from build123d import *

# Parameters (mm, degrees)
SKETCH1_W           = 30.5
SKETCH1_H           = 85
BOSS_EXTRUDE1_DEPTH = 2
CUT_EXTRUDE1_DEPTH  = 2
SKETCH5_W           = 0.8
SKETCH5_H           = 4
BOSS_EXTRUDE2_DEPTH = 3
SKETCH6_R           = 1
CUT_EXTRUDE2_DEPTH  = 0.8
FILLET1_R           = 2
FILLET2_R           = 2
SKETCH7_W           = 30.5
SKETCH7_H           = 2
BOSS_EXTRUDE3_DEPTH = 16
SKETCH8_W           = 30.5
SKETCH8_H           = 80
BOSS_EXTRUDE4_DEPTH = 1.8
SKETCH9_W           = 28.5
SKETCH9_H           = 80
CUT_EXTRUDE3_DEPTH  = 1.8
SKETCH10_W          = 28.9
SKETCH10_H          = 2
CUT_EXTRUDE4_DEPTH  = 1
SKETCH11_W          = 7
SKETCH11_H          = 6
CUT_EXTRUDE5_DEPTH  = 2


with BuildPart() as part:
    # Sketch1 → Boss-Extrude1 (new body)
    with BuildSketch(Plane(origin=(0, 0, 0), x_dir=(1, 0, 0), z_dir=(0, 1, 0))):
        Rectangle(SKETCH1_W, SKETCH1_H)
    extrude(amount=BOSS_EXTRUDE1_DEPTH)

    # Sketch2 → Cut-Extrude1 (cut)
    with BuildSketch(Plane(origin=(0, 2, 0), x_dir=(1, 0, 0), z_dir=(0, 1, 0))):
        Polygon((14.45, 42.5), (-14.45, 42.5), (-14.45, 24.5), (-14.45, 22.5), (14.45, 22.5), (14.45, 24.5), align=None)
    extrude(amount=-CUT_EXTRUDE1_DEPTH, mode=Mode.SUBTRACT)

    # Sketch5 → Boss-Extrude2 (add)
    with BuildSketch(Plane(origin=(0, 2, 0), x_dir=(1, 0, 0), z_dir=(0, 1, 0))):
        with Locations((-14.85, 40.5)):
            Rectangle(SKETCH5_W, SKETCH5_H)
    boss_extrude2 = extrude(amount=BOSS_EXTRUDE2_DEPTH)

    # Sketch6 → Cut-Extrude2 (cut)
    with BuildSketch(Plane.ZY.offset(15.25)):
        with Locations((-40.5, 2)):
            Circle(SKETCH6_R)
    cut_extrude2 = extrude(amount=-CUT_EXTRUDE2_DEPTH, mode=Mode.SUBTRACT)

    # Mirror1: Boss-Extrude2, Cut-Extrude2 across plane
    add(boss_extrude2.mirror(Plane(origin=(0, 0, 0), x_dir=(0, 0, 1), z_dir=(1, 0, 0))))
    add(cut_extrude2.mirror(Plane(origin=(0, 0, 0), x_dir=(0, 0, 1), z_dir=(1, 0, 0))), mode=Mode.SUBTRACT)

    # Fillet1
    fillet1_edges = [part.edges().sort_by_distance(p)[0] for p in [
        (-14.85, 0, -42.5),
        (-14.85, 5, -42.5),
        (-14.85, 5, -38.5),
    ]]
    fillet(fillet1_edges, radius=FILLET1_R - 0.0001)  # a hair under: the kernel refuses the full size

    # Fillet2
    fillet2_edges = [part.edges().sort_by_distance(p)[0] for p in [
        (14.85, 0, -42.5),
        (14.85, 5, -38.5),
        (14.85, 5, -42.5),
    ]]
    fillet(fillet2_edges, radius=FILLET2_R - 0.0001)  # a hair under: the kernel refuses the full size

    # Sketch7 → Boss-Extrude3 (add)
    with BuildSketch(Plane.XY.offset(42.5)):
        with Locations((0, 1)):
            Rectangle(SKETCH7_W, SKETCH7_H)
    extrude(amount=BOSS_EXTRUDE3_DEPTH)

    # Sketch8 → Boss-Extrude4 (add)
    with BuildSketch(Plane(origin=(0, 2, 0), x_dir=(1, 0, 0), z_dir=(0, 1, 0))):
        with Locations((0, -18.5)):
            Rectangle(SKETCH8_W, SKETCH8_H)
    extrude(amount=BOSS_EXTRUDE4_DEPTH)

    # Sketch9 → Cut-Extrude3 (cut)
    with BuildSketch(Plane(origin=(0, 3.8, 0), x_dir=(1, 0, 0), z_dir=(0, 1, 0))):
        with Locations((0, -18.5)):
            Rectangle(SKETCH9_W, SKETCH9_H)
    extrude(amount=-CUT_EXTRUDE3_DEPTH, mode=Mode.SUBTRACT)

    # Sketch10 → Cut-Extrude4 (cut)
    with BuildSketch(Plane(origin=(0, 0, -22.5), x_dir=(-1, 0, 0), z_dir=(0, 0, -1))):
        with Locations((0, 1)):
            Rectangle(SKETCH10_W, SKETCH10_H)
    extrude(amount=-CUT_EXTRUDE4_DEPTH, mode=Mode.SUBTRACT)

    # Sketch11 → Cut-Extrude5 (cut)
    with BuildSketch(Plane(origin=(0, 2, 0), x_dir=(1, 0, 0), z_dir=(0, 1, 0))):
        with Locations((10.75, -50.5)):
            Rectangle(SKETCH11_W, SKETCH11_H)
    extrude(amount=-CUT_EXTRUDE5_DEPTH, mode=Mode.SUBTRACT)


solid = part.part
For this review, take the finished solid that the model builds, in its own axes (mm). A direction names the side the tool comes from. Give positions to 0.01 mm unless a question says otherwise; leave off trailing zeros. Order: outer loops, then holes, each group sorted by start corner. A loop starts at its lowest first (then second) coordinate and runs counter-clockwise, first axis right, second up. Notation, with made-up numbers: (8.25, -33.5) - (25.25, -33.5) arc R20 cw to (25.25, -12.5) - close; hole circle Ø3 at (23, 2). An arc over 180 degrees is marked (long way). Answer as a JSON object with one key per item and string values. Group by question number.
Item 1: Clearance check with flat-ended pins moving along their axes: pin 1 Ø1.6 at (x, y) = (10, 1.5) entering from -Z; pin 2 Ø0.8 at (x, z) = (14.5, 29) entering from +Y; pin 3 Ø3 at (x, z) = (12, 5) entering from -Y; pin 4 Ø1.6 at (y, z) = (2, -40.5) entering from -X. State where each tip first meets the part, or that it passes through.
Item 2: Take a section at C-C on x = 1.5. Give the boundary of the cut face in (y, z), and give its area (3 significant figures).
Item 3: Draft analysis for pull direction Z (two halves, no side actions). For faces 1 (the flat face through (0, 2, 18)), 2 (the cylindrical face through (-14.84, 4.4, -39.07)), 3 (the cylindrical face through (-14.84, 0.57, -41.9)), 4 (the flat face through (11, 1, 53.5)), state which applies: pulls with the +Z half, pulls with the -Z half, needs draft (parallel to the pull), parting line crosses it, or undercut.
Item 4: Machinability: for faces 5 (the flat face through (-14.25, 3, 19)), 6 (the flat face through (15.25, 2, 9)), 7 (the flat face through (11, 1, 47.5)), 8 (the flat face through (-14.45, 1, -32)), which of the approach directions +Z, -Z, +X, -X, +Y, -Y give a long, thin tool a straight path to every point of the face, cutting with its end or side? Answer none if there is none.
Item 5: Take a section at B-B on z = -3. Give the boundary of the cut face in (x, y), and give its area (3 significant figures).
Item 6: Take a section at A-A on z = -31.5. Give the boundary of the cut face in (x, y).
Item 7: Wall thickness on line 1 along Y through (x, z) = (-14.8, -40.5); line 2 along X through (y, z) = (2.35, 31); line 3 along Z through (x, y) = (14, 0.2): over which ranges is each line inside the solid? List them lowest first.
Reported:
{
 "1": {"pin 1": "z = -21.5", "pin 2": "y = 3.8", "pin 3": "y = 0", "pin 4": "through"},
 "2": {"outline": "(0, -21.5) - (2, -21.5) - (2, 58.5) - (0, 58.5) - close", "area": "160 mm^2"},
 "3": {"face 1": "needs draft", "face 2": "undercut", "face 3": "pulls with the -Z half", "face 4": "undercut"},
 "4": {"face 5": "+Z, -Z, +Y", "face 6": "+Z, -Z, +X, +Y, -Y", "face 7": "+Y, -Y", "face 8": "-Z, +Y, -Y"},
 "5": {"outline": "(-15.25, 0) - (15.25, 0) - (15.25, 3.8) - (14.25, 3.8) - (14.25, 2) - (-14.25, 2) - (-14.25, 3.8) - (-15.25, 3.8) - close", "area": "64.6 mm^2"},
 "6": {"outline": "(-15.25, 0) - (-14.45, 0) - (-14.45, 2) - (-15.25, 2) - close; (14.45, 0) - (15.25, 0) - (15.25, 2) - (14.45, 2) - close"},
 "7": {"line 1": "0 to 1, 3 to 5", "line 2": "-15.25 to -14.25, 14.25 to 15.25", "line 3": "-21.5 to 47.5, 53.5 to 58.5"}
}
